```python
from build123d import *

# Parameters (mm, degrees)
F0_R     = 1.4732
F0_R_2   = 2.38125
F0_W     = 1.5875
F0_H     = 20
F0_W_2   = 10
F0_H_2   = 1.5875
F0_W_3   = 20
F1_DEPTH = 1.5875
F2_SIZE  = 5


# Not quite as in the source:
# - a length typed as a fraction of an inch, garbled in the dataset ("3 / 203.2 mm" for 3/8 in), is restored


with BuildPart() as f1:
    # F0 (on Front) → F1 (new body)
    with BuildSketch(Plane.XZ):
        Polygon((100, 10), (100, 25), (-100, 25), (-100, 10), (-100, -10), (-100, -25), (-90, -25), (-80, -25), (-60, -25), (-44.45, -25), (-44.45, -12.3), (-44.45, 13.1), (0, 13.1), (0, -12.3), (0, -25), (20, -25), (40, -25), (60, -25), (80, -25), (90, -25), (100, -25), (100, -10), align=None)
        with Locations((-80, 18.6)):
            Circle(F0_R, mode=Mode.SUBTRACT)
        with Locations((-64.3028, 18.6)):
            Circle(F0_R, mode=Mode.SUBTRACT)
        with Locations((55.55, 2.5678405073)):
            Circle(F0_R_2, mode=Mode.SUBTRACT)
        with Locations((74.6, 2.6706890203)):
            Circle(F0_R_2, mode=Mode.SUBTRACT)
        with Locations((64.3028, 18.6)):
            Circle(F0_R, mode=Mode.SUBTRACT)
        with Locations((80, 18.6)):
            Circle(F0_R, mode=Mode.SUBTRACT)
        with Locations((100.79375, 0)):
            Rectangle(F0_W, F0_H)
        with Locations((-100.79375, 0)):
            Rectangle(F0_W, F0_H)
        with Locations((85, -25.79375)):
            Rectangle(F0_W_2, F0_H_2)
        with Locations((-85, -25.79375)):
            Rectangle(F0_W_2, F0_H_2)
        with Locations((50, -25.79375)):
            Rectangle(F0_W_3, F0_H_2)
        Polygon((-44.45, -25), (-60, -25), (-60, -26.5875), (-40, -26.5875), (-40, -25), align=None)
        Polygon((-44.45, -12.3), (-44.45, -25), (-40, -25), (-20, -25), (0, -25), (0, -12.3), align=None)
        Polygon((20, -26.5875), (20, -25), (0, -25), (-20, -25), (-20, -26.5875), align=None)
    extrude(amount=F1_DEPTH)

    # F2
    f2_edges = [f1.edges().sort_by_distance(p)[0] for p in [
        (-44.45, -0.79375, 13.1),
        (0, -0.79375, 13.1),
    ]]
    chamfer(f2_edges, length=F2_SIZE)


solid = f1.part
```
Work out the finished part from the listing and answer in its coordinate system (mm). A direction names the side the tool comes from. Give positions to 0.01 mm unless a question says otherwise; leave off trailing zeros. Write each loop counter-clockwise with the first axis right and the second up, starting at its lowest first coordinate (ties: lowest second). Pieces come first, ordered by that corner, then holes. Notation, with made-up numbers: (87.5, 55) - (139.5, 55) arc R26 ccw to (139.5, 90) - close; hole circle Ø6 at (83.25, -31). An arc over 180 degrees is marked (long way). Use one line per item in the form item = value.
1. For faces 1 (the face through (-1, 0, 11)), 2 (the face through (-41.92, -0.78, 10.63)), determine the directions among +Z, -Z, +X, -X, +Y, -Y from which every point of the face is accessible in a straight line to the end or side of a thin tool.
Filled in:
face_1 = +Z, -Z, +X, -X, +Y
face_2 = +Y, -Y
2. A cutting plane is placed at D-D (x = 28.5). Write down the section's boundary in (y, z), and give its area (3 significant figures).
Filled in:
outline = (-1.59, -25) - (0, -25) - (0, 25) - (-1.59, 25) - close
area = 79.4 mm^2
3. Each of these flat-tipped pins is pushed along its axis until it touches: pin 1 Ø0.5 at (y, z) = (-0.5, -25.5) entering from -X; pin 2 Ø1.8 at (x, z) = (80, 18.6) entering from -Y; pin 3 Ø0.5 at (y, z) = (-0.5, -25.5) entering from +X; pin 4 Ø0.5 at (y, z) = (-0.5, -19) entering from +X. Where does it stop, or does it pass through?
Filled in:
pin_1 = -90
pin_2 = through
pin_3 = 90
pin_4 = 100
4. A cutting plane is placed at A-A (x = 55.55). Write down the section's boundary in (y, z), and give its area (3 significant figures).
Filled in:
outline = (-1.59, -26.59) - (0, -26.59) - (0, 0.19) - (-1.59, 0.19) - close; (-1.59, 4.95) - (0, 4.95) - (0, 25) - (-1.59, 25) - close
area = 74.3 mm^2
5. Determine the mould class of faces 3 (the face through (72.22, -0.78, 2.78)), 4 (the face through (-1, -1.588, 11)) for opening direction X: released by +X, released by -X, zero draft, split by the parting line, or undercut.
Filled in:
face_3 = undercut
face_4 = zero draft
6. Consider L1, parallel to X at y = -0.1, z = -5; L2, parallel to Z at x = -37.5, y = -0.3; L3, parallel to Z at x = 74.6, y = -0.95. Determine where each line is inside the solid, lowest interval first.
Filled in:
L1 = -101.59 to -44.45, 0 to 101.59
L2 = -25 to -12.3, 13.1 to 25
L3 = -25 to 0.29, 5.05 to 25
7. A cutting plane is placed at B-B (z = -4). Write down the section's boundary in (x, y).
Filled in:
outline = (-101.59, -1.59) - (-44.45, -1.59) - (-44.45, 0) - (-101.59, 0) - close; (0, -1.59) - (101.59, -1.59) - (101.59, 0) - (0, 0) - close
8. A cutting plane is placed at C-C (y = -1.1). State how many separate pieces and enclosed holes the cut face has, and give its area (3 significant figures).
Filled in:
separate_pieces = 1
enclosed_holes = 7
area = 9,060 mm^2
